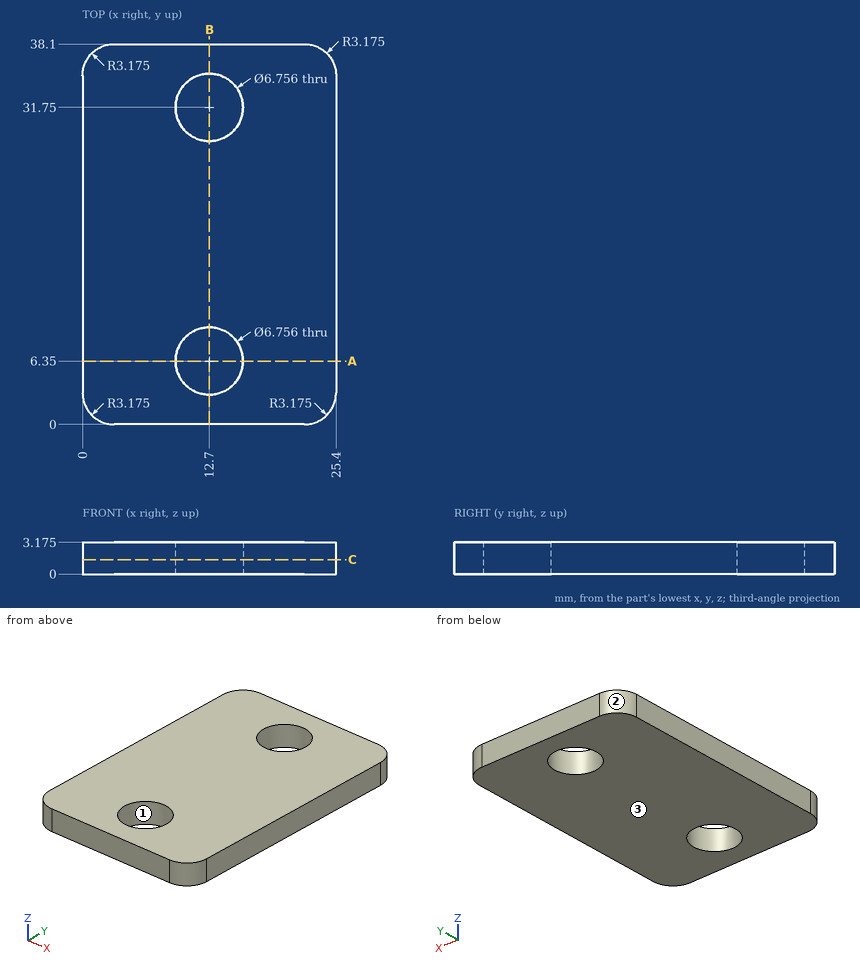
Geometry check sheet. Reference: drawing and pictorial views, mm from the part's lowest x, y, z. Give positions to 0.01 mm unless a question says otherwise; leave off trailing zeros. Write each loop counter-clockwise with the first axis right and the second up, starting at its lowest first coordinate (ties: lowest second). Pieces come first, ordered by that corner, then holes. Notation, with made-up numbers: (4.25, 58.5) - (47.25, 58.5) arc R19 cw to (47.25, 89.5) - close; hole circle Ø5 at (4, 76.5). An arc over 180 degrees is marked (long way). Use a Markdown table: item, result.
Q1. Section check B-B, the plane x = 12.7. Enter the section's corners in (y, z) (1 decimal).
Computed:
| item | result |
|---|---|
| outline | (0, 0) - (3, 0) - (3, 3.2) - (0, 3.2) - close; (9.7, 0) - (28.4, 0) - (28.4, 3.2) - (9.7, 3.2) - close; (35.1, 0) - (38.1, 0) - (38.1, 3.2) - (35.1, 3.2) - close |
Q2. Section check A-A, the plane y = 6.35. Enter the section's corners in (x, z) (1 decimal).
Computed:
| item | result |
|---|---|
| outline | (0, 0) - (9.3, 0) - (9.3, 3.2) - (0, 3.2) - close; (16.1, 0) - (25.4, 0) - (25.4, 3.2) - (16.1, 3.2) - close |
Q3. Thickness scan on L1, parallel to Y at x = 12.7, z = 2.3; L2, parallel to Y at x = 11.5, z = 0.2; L3, parallel to X at y = 5.5, z = 0.8. Record the ranges inside material, lowest first. Write a range as [from, to].
Computed:
| item | result |
|---|---|
| L1 | y = [0, 2.97], [9.73, 28.37], [35.13, 38.1] |
| L2 | y = [0, 3.19], [9.51, 28.59], [34.91, 38.1] |
| L3 | x = [0, 9.43], [15.97, 25.4] |
Q4. Section check C-C, the plane z = 1.45. Give the number of separate pieces and of enclosed holes in the cut face.
Computed:
| item | result |
|---|---|
| separate pieces | 1 |
| enclosed holes | 2 |
Q5. Draft check along X on the marked faces 1, 2 and 3. Enter one of: pulls with the +X half, pulls with the -X half, needs draft (parallel to the pull), parting line crosses it, or undercut.
Computed:
| item | result |
|---|---|
| face 1 | undercut |
| face 2 | pulls with the -X half |
| face 3 | needs draft |
